Geometry check sheet. Reference: the model listing, model coordinates, mm. Face numbers are marked on the shaded views. A direction names the side the tool comes from. Round coordinates to 2 decimals unless told otherwise and drop trailing zeros. Order: outer loops, then holes, each group sorted by start corner. A loop starts at its lowest first (then second) coordinate and runs counter-clockwise, first axis right, second up. Notation, with made-up numbers: (78.5, 40.25) -> (109.5, 40.25) arc R11 ccw to (109.5, 46.25) -> close; hole circle Ø5 at (82.25, -5). An arc over 180 degrees is marked (long way). Answer as a JSON object with one key per item and string values. Group by question number.
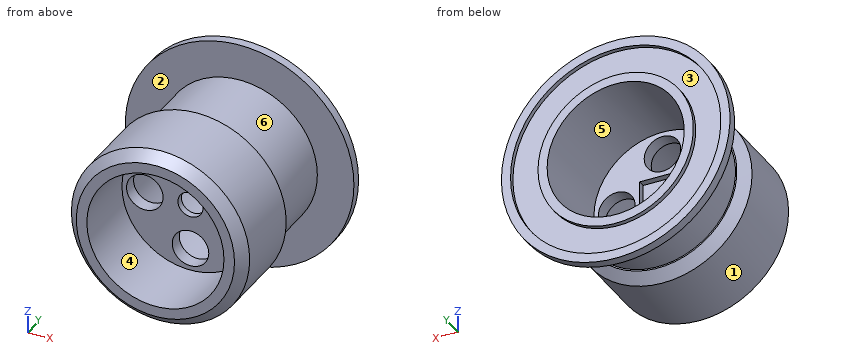
from build123d import *

# Parameters (mm, degrees)
SKETCH_3_R          = 23
SKETCH_3_R_2        = 17
CUT_EXTRUDE_1_DEPTH = 1
SKETCH_4_W          = 10
SKETCH_4_H          = 10
CUT_EXTRUDE_2_DEPTH = 1.5
SKETCH_5_R          = 4
CUT_EXTRUDE_3_DEPTH = 3
SKETCH_9_R          = 17
SKETCH_9_R_2        = 4
EXTRUDE_1_DEPTH     = 1
SKETCH_10_R         = 17
SKETCH_10_R_2       = 15
EXTRUDE_2_DEPTH     = 15
SKETCH_11_R         = 2.75
CUT_EXTRUDE_4_DEPTH = 17.5
SKETCH_12_R         = 19.5
SKETCH_12_R_2       = 17
EXTRUDE_3_DEPTH     = 20
CHAMFER_1_SIZE      = 2.195


with BuildPart() as part:
    # Эскиз2 → Повернуть1 (revolve)
    with BuildSketch(Plane.XY):
        Polygon((15, 0), (15, -20), (0, -20), (0, -22), (17, -22), (17, -2), (25, -2), (25, 0), align=None)
    revolve(axis=Axis((0, 0, 0), (0, -1, 0)))

    # Эскиз3 → Вырез-Вытянуть1 (cut)
    with BuildSketch(Plane(origin=(0, 0, 0), x_dir=(1, 0, 0), z_dir=(0, 1, 0))):
        Circle(SKETCH_3_R)
        Circle(SKETCH_3_R_2, mode=Mode.SUBTRACT)
    extrude(amount=-CUT_EXTRUDE_1_DEPTH, mode=Mode.SUBTRACT)

    # Эскиз4 → Вырез-Вытянуть2 (cut)
    with BuildSketch(Plane(origin=(0, -20, 0), x_dir=(1, 0, 0), z_dir=(0, 1, 0))):
        Rectangle(SKETCH_4_W, SKETCH_4_H)
    extrude(amount=-CUT_EXTRUDE_2_DEPTH, mode=Mode.SUBTRACT)

    # Эскиз5 → Вырез-Вытянуть3 (cut, through all)
    with BuildSketch(Plane(origin=(0, -20, 0), x_dir=(1, 0, 0), z_dir=(0, 1, 0))):
        with Locations((0, 10)):
            Circle(SKETCH_5_R)
        with Locations((10, 0)):
            Circle(SKETCH_5_R)
        with Locations((0, -10)):
            Circle(SKETCH_5_R)
        with Locations((-10, 0)):
            Circle(SKETCH_5_R)
    extrude(amount=-CUT_EXTRUDE_3_DEPTH, mode=Mode.SUBTRACT)

    # Эскиз9 → Бобышка-Вытянуть1 (add)
    with BuildSketch(Plane.XZ.offset(22)):
        Circle(SKETCH_9_R)
        with Locations((0, 10)):
            Circle(SKETCH_9_R_2, mode=Mode.SUBTRACT)
        with Locations((-10, 0)):
            Circle(SKETCH_9_R_2, mode=Mode.SUBTRACT)
        with Locations((0, -10)):
            Circle(SKETCH_9_R_2, mode=Mode.SUBTRACT)
        with Locations((10, 0)):
            Circle(SKETCH_9_R_2, mode=Mode.SUBTRACT)
    extrude(amount=EXTRUDE_1_DEPTH)

    # Эскиз10 → Бобышка-Вытянуть2 (add)
    with BuildSketch(Plane.XZ.offset(23)):
        Circle(SKETCH_10_R)
        Circle(SKETCH_10_R_2, mode=Mode.SUBTRACT)
    extrude(amount=EXTRUDE_2_DEPTH)

    # Эскиз11 → Вырез-Вытянуть4 (cut, through all)
    with BuildSketch(Plane(origin=(0, -21.5, 0), x_dir=(1, 0, 0), z_dir=(0, 1, 0))):
        Circle(SKETCH_11_R)
    extrude(amount=-CUT_EXTRUDE_4_DEPTH, mode=Mode.SUBTRACT)

    # Эскиз12 → Бобышка-Вытянуть3 (add)
    with BuildSketch(Plane.XZ.offset(38)):
        Circle(SKETCH_12_R)
        Circle(SKETCH_12_R_2, mode=Mode.SUBTRACT)
    extrude(amount=-EXTRUDE_3_DEPTH)

    # Фаска1
    chamfer_1_edges = [part.edges().sort_by_distance(p)[0] for p in [
        (-19.5, -18, 0),
        (-19.5, -38, 0),
    ]]
    chamfer(chamfer_1_edges, length=CHAMFER_1_SIZE)


solid = part.part
Item 1: Mould release check, pull along Y, two halves, no side actions. Record for the marked faces 1, 2 and 3: pulls with the +Y half, pulls with the -Y half, needs draft (parallel to the pull), parting line crosses it, or undercut.
Item 2: Set-up check for the marked faces 4, 5 and 6: record each of +Z, -Z, +X, -X, +Y, -Y from which the full face is reachable in a straight line by a thin tool's end or side.
Item 3: Depth check by flat-ended pin: pin 1 Ø5 at (x, y) = (17.5, -25.5) entering from -Z; pin 2 Ø8 at (y, z) = (-28.5, -15) entering from -X; pin 3 Ø3 at (x, y) = (-0.5, -10.5) entering from -Z. Enter the tip coordinate at first touch or a pass-through.
Item 4: Sectioned sample at A-A, the plane z = 0. Count the separate pieces of the cut face and the enclosed holes in it, then the cut area to 3 significant figures.
Item 5: Thickness scan on L1, parallel to Y at x = -6, z = -0.5; L2, parallel to Z at x = 11, y = -2.5; L3, parallel to Z at x = -11.5, y = -36. Record the ranges inside material, lowest first.
Item 6: Sectioned sample at C-C, the plane x = 20.5. Enter the section's corners in (y, z), then the cut area to 3 significant figures.
Item 7: Sectioned sample at D-D, the plane z = -21.5. Enter the section's corners in (x, y).
Result:
{
 "1": {"face 1": "needs draft", "face 2": "undercut", "face 3": "pulls with the +Y half"},
 "2": {"face 4": "-Y", "face 5": "+Y", "face 6": "none"},
 "3": {"pin 1": "stops at z = -12.46", "pin 2": "stops at x = -16.1", "pin 3": "stops at z = -17"},
 "4": {"separate pieces": "4", "enclosed holes": "0", "area": "281 mm2"},
 "5": {"L1": "y = -23 to -20", "L2": "z = -12.96 to -10.2, 10.2 to 12.96", "L3": "z = -15.51 to -9.63, 9.63 to 15.51"},
 "6": {"outline": "(-2, -14.31) -> (0, -14.31) -> (0, -10.43) -> (-1, -10.43) -> (-1, 10.43) -> (0, 10.43) -> (0, 14.31) -> (-2, 14.31) -> close", "area": "36.4 mm2"},
 "7": {"outline": "(-12.76, -2) -> (12.76, -2) -> (12.76, 0) -> (8.17, 0) -> (8.17, -1) -> (-8.17, -1) -> (-8.17, 0) -> (-12.76, 0) -> close"}
}
